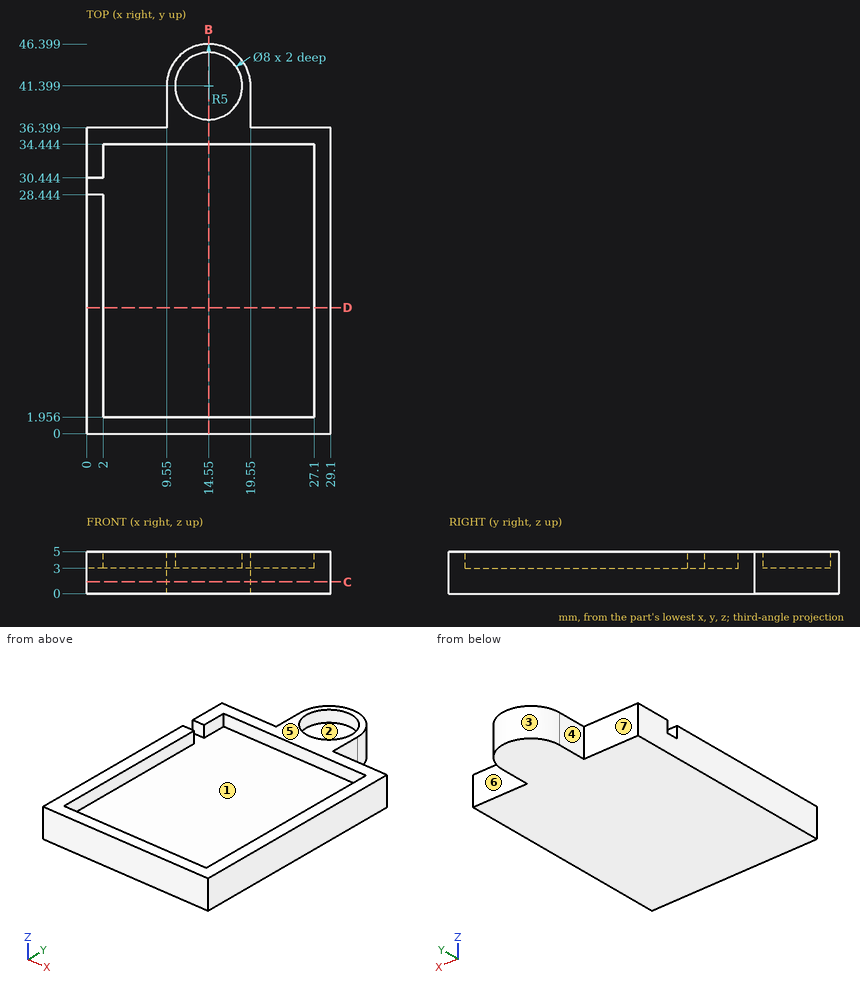
Design review of the part shown in the three views and the two pictorial views. Dimensions are in mm from the part's minimum x, y and z. A direction names the side the tool comes from. Round coordinates to 2 decimals unless told otherwise and drop trailing zeros. Loops run counter-clockwise (first coordinate to the right, second up) from the corner with the lowest first, then second, coordinate; pieces in that order, holes last. Notation, with made-up numbers: (-16.75, -34.5) -> (-0.75, -34.5) arc R28 ccw to (-0.75, -6.5) -> close; hole circle Ø1 at (33, 19). An arc over 180 degrees is marked (long way). Use one line per item in the form item = value. Start each with the question number.
Q1. Wall thickness on line 1 along Y through (x, z) = (14.55, 3.9) (1 decimal); line 2 along Y through (x, z) = (5.75, 3.8) (1 decimal); line 3 along X through (y, z) = (31, 3.6): over which ranges is each line inside the solid? List them lowest first. Write a range as [from, to].
Q2. We need section B-B on x = 14.55. Give the boundary of the cut face in (y, z) (1 decimal), then the cut area to 3 significant figures.
Q3. Machinability: for the marked faces 5, 6 and 7, which of the approach directions +Z, -Z, +X, -X, +Y, -Y give a long, thin tool a straight path to every point of the face, cutting with its end or side? Answer none if there is none.
Q4. For pin 1 Ø9 at (x, y) = (14.55, 41.4) entering from -Z; pin 2 Ø1.6 at (x, z) = (1.5, 4) entering from +Y; pin 3 Ø2.5 at (x, y) = (16.5, 40.5) entering from +Z; pin 4 Ø1 at (x, z) = (13.5, 4.5) entering from +Y, all flat-tipped, find the tip position at first contact; note any pin that passes through.
Q5. Draft analysis for pull direction X (two halves, no side actions). For the marked faces 1, 2, 3 and 4, state which applies: +X half, -X half, draft (parallel to the pull), parting line (faces both ways), or undercut.
Q6. We need section C-C on z = 1.4. Give the boundary of the cut face in (x, y).
Q7. We need section D-D on y = 15. Give the boundary of the cut face in (x, z).
Calculated:
q1.line_1 = [0, 2], [34.4, 37.4], [45.4, 46.4]
q1.line_2 = [0, 2], [34.4, 36.4]
q1.line_3 = [0, 2], [27.1, 29.1]
q2.outline = (0, 0) -> (46.4, 0) -> (46.4, 5) -> (45.4, 5) -> (45.4, 3) -> (37.4, 3) -> (37.4, 5) -> (34.4, 5) -> (34.4, 3) -> (2, 3) -> (2, 5) -> (0, 5) -> close
q2.area = 151 mm²
q3.face_5 = +Z, +X, -X, +Y, -Y
q3.face_6 = +Z, -Z, +X, +Y
q3.face_7 = +Z, -Z, -X, +Y
q4.pin_1 = 0
q4.pin_2 = 36.4
q4.pin_3 = 3
q4.pin_4 = 46.37
q5.face_1 = undercut
q5.face_2 = undercut
q5.face_3 = parting line
q5.face_4 = -X half
q6.outline = (0, 0) -> (29.1, 0) -> (29.1, 36.4) -> (19.55, 36.4) -> (19.55, 41.4) arc R5 ccw to (9.55, 41.4) -> (9.55, 36.4) -> (0, 36.4) -> close
q7.outline = (0, 0) -> (29.1, 0) -> (29.1, 5) -> (27.1, 5) -> (27.1, 3) -> (2, 3) -> (2, 5) -> (0, 5) -> close
